Geometry check sheet. Reference: drawing and pictorial views, mm from the part's lowest x, y, z. A direction names the side the tool comes from. Round coordinates to 2 decimals unless told otherwise and drop trailing zeros. Write each loop counter-clockwise with the first axis right and the second up, starting at its lowest first coordinate (ties: lowest second). Pieces come first, ordered by that corner, then holes. Notation, with made-up numbers: (87, 75.5) - (112, 75.5) arc R15 cw to (112, 90.5) - close; hole circle Ø4 at (45, -23). An arc over 180 degrees is marked (long way). Use one line per item in the form item = value. Start each with the question number.
1) Section check C-C (z = 30). Record the boundary of the cut face in (x, y).
2) Gauge pin test, flat ends, axial feed: P1, Ø14.5, axis at x = 22, z = 33, coming from the -Y side; P2, Ø24, axis at y = 8, z = 21.5, coming from the -X side. Record the tip position at first contact, or that the pin passes through.
3) Section check B-B (x = 12). Record the boundary of the cut face in (y, z), then the cut area to 3 significant figures.
4) Set-up check for the marked faces 1, 2 and 3: record each of +Z, -Z, +X, -X, +Y, -Y from which the full face is reachable in a straight line by a thin tool's end or side.
5) Section check A-A (y = 43.5). Record the boundary of the cut face in (x, z).
6) Scan lines: probe 1 along Y at (x, z) = (16.5, 54.5); probe 2 along X at (y, z) = (29, 64). Record each from-to range of solid material in increasing order.
7) Draft check along Y on the marked faces 4, 5 and 6. Enter one of: +Y half, -Y half, draft (parallel to the pull), parting line (faces both ways), or undercut.
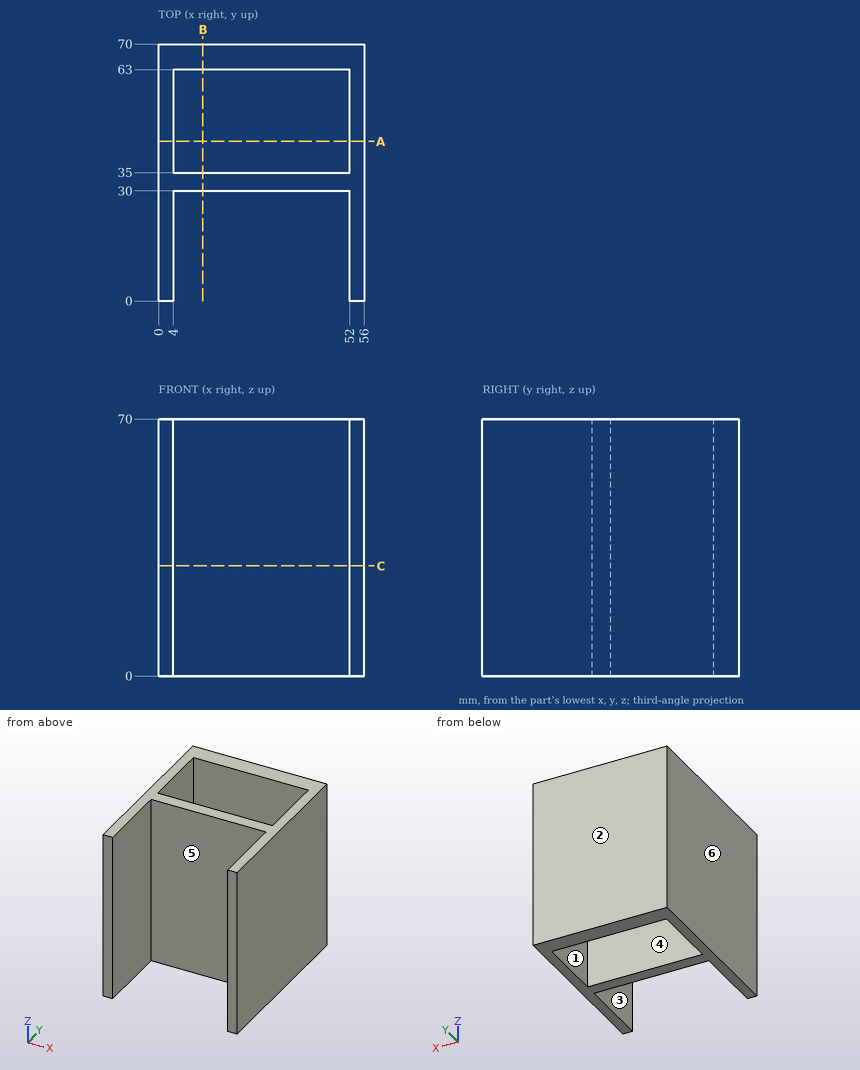
Results are:
q1.outline = (0, 0) - (4, 0) - (4, 30) - (52, 30) - (52, 0) - (56, 0) - (56, 70) - (0, 70) - close; hole (4, 35) - (52, 35) - (52, 63) - (4, 63) - close
q2.P1 = 30
q2.P2 = 0
q3.outline = (30, 0) - (35, 0) - (35, 70) - (30, 70) - close; (63, 0) - (70, 0) - (70, 70) - (63, 70) - close
q3.area = 840 mm²
q4.face_1 = +Z, -Z
q4.face_2 = +Z, -Z, +X, -X, +Y
q4.face_3 = +Z, -Z, -Y
q5.outline = (0, 0) - (4, 0) - (4, 70) - (0, 70) - close; (52, 0) - (56, 0) - (56, 70) - (52, 70) - close
q6.probe_1 = 30 to 35, 63 to 70
q6.probe_2 = 0 to 4, 52 to 56
q7.face_4 = undercut
q7.face_5 = -Y half
q7.face_6 = draft
